Autodesk Inventor part; units mm, degrees
ref_plane "YZ Plane" through (0, 0, 0) normal (1, 0, 0) x (0, 1, 0)
ref_plane "XZ Plane" through (0, 0, 0) normal (0, 1, 0) x (-1, 0, 0)
ref_plane "XY Plane" through (0, 0, 0) normal (0, 0, 1) x (1, 0, 0)
sketch "Sketch5" plane through (0, 0, 0) normal (0, 0, 1) x (1, 0, 0)
  line L0 (0, 0) -> (82.55, 0)
  line L1 (82.55, 0) -> (82.55, 38.1)
  line L2 (82.55, 38.1) -> (0, 38.1)
  line L3 (0, 38.1) -> (0, 0)
  dimension "d41" = 82.55
  dimension "d42" = 38.1
extrude "Extrusion5" add sketch "Sketch5" along normal blind 3.175
sketch "Sketch6" plane through (0, 0, 3.175) normal (0, 0, 1) x (1, 0, 0)
  line L0 (0, 0) -> (82.55, 0)
  line L1 (82.55, 0) -> (82.55, 38.1)
  line L2 (82.55, 38.1) -> (0, 38.1)
  line L3 (0, 38.1) -> (0, 0)
  line L4 (0, 38.1) -> (0, 0)
  line L5 (79.375, 3.175) -> (79.375, 9.525)
  line L6 (79.375, 9.525) -> (76.2, 9.525)
  line L7 (76.2, 9.525) -> (76.2, 3.175)
  line L8 (3.175, 3.175) -> (3.175, 9.525)
  line L9 (3.175, 9.525) -> (6.35, 9.525)
  line L10 (6.35, 9.525) -> (6.35, 3.175)
  line L11 (6.35, 3.175) -> (9.525, 3.175)
  line L12 (9.525, 3.175) -> (9.525, 12.7)
  line L13 (9.525, 12.7) -> (3.175, 12.7)
  line L14 (3.175, 12.7) -> (3.175, 34.925)
  line L15 (3.175, 34.925) -> (79.375, 34.925)
  line L16 (79.375, 34.925) -> (79.375, 12.7)
  line L17 (79.375, 12.7) -> (73.025, 12.7)
  line L18 (73.025, 12.7) -> (73.025, 3.175)
  line L19 (6.35, 3.175) -> (9.525, 3.175)
  line L20 (73.025, 3.175) -> (76.2, 3.175)
  line L21 (0, 38.1) -> (82.55, 38.1)
  line L22 (82.55, 38.1) -> (82.55, 0)
  line L23 (0, 0) -> (0, 38.1)
  line L24 (82.55, 0) -> (82.55, 3.175)
  line L25 (82.55, 0) -> (82.55, 38.1)
  line L26 (82.55, 3.175) -> (79.375, 3.175)
  line L27 (0, 0) -> (0, 3.175)
  line L28 (0, 3.175) -> (3.175, 3.175)
  point P0 (3.175, 0)
  dimension "d47" = 6.35
  dimension "d48" = 3.175
  dimension "d51" = 3.175
  dimension "d52" = 3.175
  dimension "d53" = 9.525
  dimension "d54" = 6.35
  dimension "d55" = 22.225
  dimension "d56" = 6.35
  dimension "d61" = 3.175
  dimension "d62" = 3.175
extrude "Extrusion7" add sketch "Sketch6" along normal blind 87.5792 contours L3 L2 L1 L26 L5 L6 L7 L20 L18 L17 L16 L15 L14 L13 L12 L11 L10 L9 L8 L28
sketch "Sketch7" plane through (0, 0, 0) normal (0, 0, -1) x (-1, 0, 0)
  line L0 (0, 0) -> (0, 22.225)
  line L1 (0, 38.1) -> (0, 0)
  line L2 (0, 22.225) -> (-82.55, 22.225)
  line L3 (-82.55, 0) -> (-82.55, 38.1)
  line L4 (-82.55, 22.225) -> (0, 22.225)
  line L5 (0, 22.225) -> (0, 38.1)
  line L6 (0, 38.1) -> (-82.55, 38.1)
  line L7 (-82.55, 38.1) -> (-82.55, 22.225)
  dimension "d63" = 22.225
extrude "Extrusion8" cut sketch "Sketch7" against normal up to next
sketch "Sketch8" plane through (0, 22.225, 0) normal (0, 1, 0) x (1, 0, 0)
  line L0 (0, 0) -> (82.55, 0)
  line L1 (0, 0) -> (82.55, 0)
  line L2 (82.55, -104.775) -> (0, -104.775)
  line L3 (0, -104.775) -> (0, 0)
  line L4 (82.55, 0) -> (82.55, -104.775)
  dimension "d66" = 104.775
extrude "Extrusion9" add sketch "Sketch8" along normal blind 3.175
chamfer "Chamfer2" distance 12.7 angle 45 2 edges at (82.55, 23.8125, 104.775) (0, 23.8125, 104.775)
properties part number "top-slider"
The model under review builds one solid part; all positions refer to its coordinate system, in mm. A direction names the side the tool comes from. Round coordinates to 2 decimals unless told otherwise and drop trailing zeros. Loops run counter-clockwise (first coordinate to the right, second up) from the corner with the lowest first, then second, coordinate; pieces in that order, holes last. Notation, with made-up numbers: (3.5, -2.75) - (14.5, -2.75) arc R26 ccw to (14.5, 34.25) - close; hole circle Ø6 at (21.25, -5.75). An arc over 180 degrees is marked (long way). Use a Markdown table: item, result. Add a question column.
Q1. Add section A-A (z = 67.5). State the section outline as (x, y) points (3 decimals), plus the area to 3 significant figures.
Q2. Add section B-B (y = 16.5). State the section outline as (x, z) points (3 decimals).
Q3. The part is to be moulded in two halves that separate along X. For faces 4 (the face through (4, 11, 90.754)), 5 (the face through (76.111, 23.79, 98.514)), 6 (the face through (6, 12.7, 46)), say which applies: pulls with the +X half, pulls with the -X half, needs draft (parallel to the pull), parting line crosses it, or undercut.
Q4. Machinability: for faces 1 (the face through (8, 3.175, 46)), 2 (the face through (41, 13, 0)), 3 (the face through (73.025, 8, 46)), which of the approach directions +Z, -Z, +X, -X, +Y, -Y give a long, thin tool a straight path to every point of the face, cutting with its end or side? Answer none if there is none.
Q5. For probe 1 along X at (y, z) = (4.25, 31.5) (3 decimals); probe 2 along X at (y, z) = (12.75, 25) (3 decimals); probe 3 along X at (y, z) = (11, 35) (3 decimals), list the stretches that pass through material, from the lowest coordinate up.
Q6. Add section C-C (x = 18). State the section outline as (y, z) points (3 decimals), plus the area to 3 significant figures.
Q7. Insertion check: pin 1 Ø1 at (x, z) = (1.5, 68.5) entering from -Y (3 decimals); pin 2 Ø7.5 at (x, y) = (77.5, 12) entering from +Z; pin 3 Ø1.5 at (x, z) = (15.5, 54) entering from -Y (3 decimals). Each pin has a flat end and moves straight along its axis. Give the tip position at first contact, or say it passes through.
Worked answers:
| question | item | result |
|---|---|---|
| 1 | outline | (0, 3.175) - (3.175, 3.175) - (3.175, 9.525) - (6.35, 9.525) - (6.35, 3.175) - (9.525, 3.175) - (9.525, 12.7) - (3.175, 12.7) - (3.175, 22.225) - (79.375, 22.225) - (79.375, 12.7) - (73.025, 12.7) - (73.025, 3.175) - (76.2, 3.175) - (76.2, 9.525) - (79.375, 9.525) - (79.375, 3.175) - (82.55, 3.175) - (82.55, 25.4) - (0, 25.4) - close |
| 1 | area | 464 mm² |
| 2 | outline | (0, 0) - (82.55, 0) - (82.55, 90.754) - (79.375, 90.754) - (79.375, 3.175) - (3.175, 3.175) - (3.175, 90.754) - (0, 90.754) - close |
| 3 | face 4 | needs draft |
| 3 | face 5 | pulls with the +X half |
| 3 | face 6 | undercut |
| 4 | face 1 | +Z, +X, -X, -Y |
| 4 | face 2 | -Z, +X, -X, +Y, -Y |
| 4 | face 3 | +Z, -Y |
| 5 | probe 1 | 0 to 3.175, 6.35 to 9.525, 73.025 to 76.2, 79.375 to 82.55 |
| 5 | probe 2 | 0 to 3.175, 79.375 to 82.55 |
| 5 | probe 3 | 0 to 9.525, 73.025 to 82.55 |
| 6 | outline | (0, 0) - (25.4, 0) - (25.4, 104.775) - (22.225, 104.775) - (22.225, 3.175) - (0, 3.175) - close |
| 6 | area | 403 mm² |
| 7 | pin 1 | y = 3.175 |
| 7 | pin 2 | z = 90.75 |
| 7 | pin 3 | y = 22.225 |
